Read the model definition and answer for the solid it produces. Units are mm, in the model's axes. Give positions to 0.01 mm unless a question says otherwise; leave off trailing zeros. Order: outer loops, then holes, each group sorted by start corner. A loop starts at its lowest first (then second) coordinate and runs counter-clockwise, first axis right, second up. Notation, with made-up numbers: (85.25, 55) - (127.25, 55) arc R11 ccw to (127.25, 74) - close; hole circle Ø10 at (-16.5, 33). An arc over 180 degrees is marked (long way). Return JSON: item names as keys, results as strings.
Autodesk Inventor part; units mm, degrees
ref_plane "YZ Plane" through (0, 0, 0) normal (1, 0, 0) x (0, 1, 0)
ref_plane "XZ Plane" through (0, 0, 0) normal (0, 1, 0) x (-1, 0, 0)
ref_plane "XY Plane" through (0, 0, 0) normal (0, 0, 1) x (1, 0, 0)
sketch "Sketch1" plane through (0, 0, 0) normal (0, 0, 1) x (1, 0, 0)
  circle A0 centre (0, 0) radius 4.88
  line L0 (0, 9) -> (30, 9)
  arc A1 (30, -9) -> (30, 9) centre (30, 0) ccw
  line L1 (30, -9) -> (0, -9)
  arc A2 (0, 9) -> (0, -9) centre (0, 0) ccw
  circle A3 centre (30, 0) radius 4.88
  dimension "d0" = 9.76
  dimension "d1" = 9
  dimension "d2" = 30
extrude "Extrusion1" add sketch "Sketch1" along normal blind 3.175
properties part number "tipper_link_D"
Q1. A cutting plane is placed at C-C (z = 0.7). Write down the section's boundary in (x, y), and give its area (3 significant figures).
Values:
{"outline": "(0, -9) - (30, -9) arc R9 ccw to (30, 9) - (0, 9) arc R9 ccw to start; hole circle Ø9.76 at (0, 0); hole circle Ø9.76 at (30, 0)", "area": "645 mm²"}
Q2. A cutting plane is placed at D-D (y = -2.5). Write down the section's boundary in (x, z) (3 decimals), and give its area (3 significant figures).
Values:
{"outline": "(-8.646, 0) - (-4.191, 0) - (-4.191, 3.175) - (-8.646, 3.175) - close; (4.191, 0) - (25.809, 0) - (25.809, 3.175) - (4.191, 3.175) - close; (34.191, 0) - (38.646, 0) - (38.646, 3.175) - (34.191, 3.175) - close", "area": "96.9 mm²"}
Q3. Given pin 1 (1.5 mm diameter, centred on y = -1, z = 3, fed in from -X); pin 2 (1 mm diameter, centred on y = -2, z = 2.5, fed in from +X), each flat-ended and moving along its own axis, determine where each tip first touches the part or whether it passes through.
Values:
{"pin 1": "stops at x = -9", "pin 2": "stops at x = 38.87"}
Q4. A cutting plane is placed at A-A (y = 0). Write down the section's boundary in (x, z) (3 decimals), and give its area (3 significant figures).
Values:
{"outline": "(-9, 0) - (-4.88, 0) - (-4.88, 3.175) - (-9, 3.175) - close; (4.88, 0) - (25.12, 0) - (25.12, 3.175) - (4.88, 3.175) - close; (34.88, 0) - (39, 0) - (39, 3.175) - (34.88, 3.175) - close", "area": "90.4 mm²"}
Q5. Consider L1, parallel to Y at x = 30, z = 0.9; L2, parallel to X at y = 2.5, z = 1; L3, parallel to X at y = -2.25, z = 2.3. Determine where each line is inside the solid, lowest interval first.
Values:
{"L1": "y = -9 to -4.88, 4.88 to 9", "L2": "x = -8.65 to -4.19, 4.19 to 25.81, 34.19 to 38.65", "L3": "x = -8.71 to -4.33, 4.33 to 25.67, 34.33 to 38.71"}
Q6. Determine the mould class of faces 1 (the flat face through (15, 0, 0)), 2 (the cylindrical face through (39, 0, 2)), 3 (the cylindrical face through (-1.058, 4.764, 1.565)) for opening direction X: released by +X, released by -X, zero draft, split by the parting line, or undercut.
Values:
{"face 1": "zero draft", "face 2": "released by +X", "face 3": "undercut"}
Q7. A cutting plane is placed at B-B (x = 33.5). Write down the section's boundary in (y, z) (3 decimals), and give its area (3 significant figures).
Values:
{"outline": "(-8.292, 0) - (-3.401, 0) - (-3.401, 3.175) - (-8.292, 3.175) - close; (3.401, 0) - (8.292, 0) - (8.292, 3.175) - (3.401, 3.175) - close", "area": "31.1 mm²"}
